The model under review builds one solid part; all positions refer to its coordinate system, in mm. Face numbers are marked on the shaded views. A direction names the side the tool comes from. Coordinates: 2 decimals unless noted, no trailing zeros. Order: outer loops, then holes, each group sorted by start corner. A loop starts at its lowest first (then second) coordinate and runs counter-clockwise, first axis right, second up.
```python
from build123d import *

# Parameters (mm, degrees)
BOSS_EXTRU_1_DEPTH      = 36
ESQUISSE2_W             = 20
ESQUISSE2_H             = 15
BOSS_EXTRU_2_DEPTH      = 4
ESQUISSE3_R             = 3.2
ENL_V_MAT_EXTRU_1_DEPTH = 4
ESQUISSE4_W             = 20
ESQUISSE4_H             = 4
BOSS_EXTRU_3_DEPTH      = 10


with BuildPart() as part:
    # Esquisse1 → Boss.-Extru.1 (new body)
    with BuildSketch(Plane.XY):
        Polygon((0, 0), (-5, 0), (-5, 15), (0, 15), (0, 9), (-3, 9), (-3, 6), (0, 6), (0, 2), (10, 2), (10, 6), (13, 6), (13, 9), (10, 9), (10, 15), (15, 15), (15, 0), (10, 0), align=None)
    extrude(amount=BOSS_EXTRU_1_DEPTH)

    # Esquisse2 → Boss.-Extru.2 (add)
    with BuildSketch(Plane.XY.offset(36)):
        with Locations((5, 7.5)):
            Rectangle(ESQUISSE2_W, ESQUISSE2_H)
    extrude(amount=BOSS_EXTRU_2_DEPTH)

    # Esquisse3 → Enlèv. mat.-Extru.1 (cut)
    with BuildSketch(Plane.XY.offset(40)):
        with Locations((5, 7.5)):
            Circle(ESQUISSE3_R)
    extrude(amount=-ENL_V_MAT_EXTRU_1_DEPTH, mode=Mode.SUBTRACT)

    # Esquisse4 → Boss.-Extru.3 (add)
    with BuildSketch(Plane(origin=(0, 15, 0), x_dir=(1, 0, 0), z_dir=(0, 1, 0))):
        with Locations((5, -38)):
            Rectangle(ESQUISSE4_W, ESQUISSE4_H)
    extrude(amount=BOSS_EXTRU_3_DEPTH)


solid = part.part
```
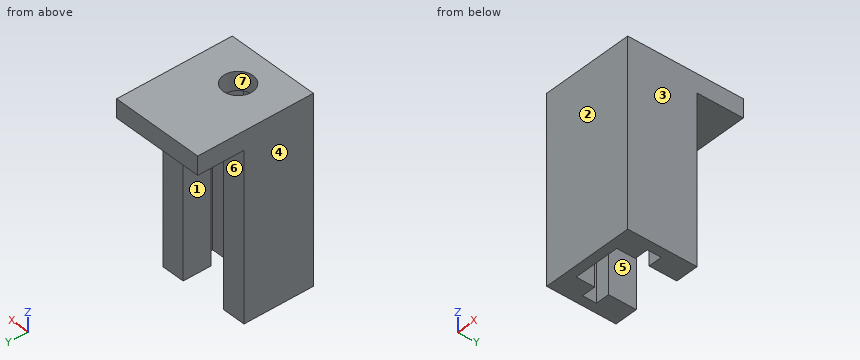
(1) Draft analysis for pull direction X (two halves, no side actions). For the marked faces 1, 2, 3 and 4, state which applies: released by +X, released by -X, zero draft, split by the parting line, or undercut.
A:
face 1: undercut
face 2: zero draft
face 3: released by +X
face 4: released by -X
(2) We need section B-B, the plane y = 7.5. Write out the cut boundary in (x, z), and give its area (3 significant figures).
A:
outline: (-5, 0) - (-3, 0) - (-3, 36) - (1.8, 36) - (1.8, 40) - (-5, 40) - close; (8.2, 36) - (13, 36) - (13, 0) - (15, 0) - (15, 40) - (8.2, 40) - close
area: 198 mm2
(3) Machinability: for the marked faces 5, 6 and 7, which of the approach directions +Z, -Z, +X, -X, +Y, -Y give a long, thin tool a straight path to every point of the face, cutting with its end or side? Answer none if there is none.
A:
face 5: -Z, +Y
face 6: -Z, +X, -X, +Y
face 7: +Z, -Z
(4) We need section D-D, the plane y = 11.75. Write out the cut boundary in (x, z).
A:
outline: (-5, 0) - (0, 0) - (0, 36) - (10, 36) - (10, 0) - (15, 0) - (15, 40) - (-5, 40) - close
(5) We need section C-C, the plane z = 28.5. Write out the cut boundary in (x, y).
A:
outline: (-5, 0) - (15, 0) - (15, 15) - (10, 15) - (10, 9) - (13, 9) - (13, 6) - (10, 6) - (10, 2) - (0, 2) - (0, 6) - (-3, 6) - (-3, 9) - (0, 9) - (0, 15) - (-5, 15) - close
(6) We need section A-A, the plane x = 5. Write out the cut boundary in (y, z).
A:
outline: (0, 0) - (2, 0) - (2, 36) - (4.3, 36) - (4.3, 40) - (0, 40) - close; (10.7, 36) - (25, 36) - (25, 40) - (10.7, 40) - close
(7) For pin 1 Ø3.5 at (x, z) = (-1, 17) entering from +Y; pin 2 Ø3 at (x, y) = (12, 19.5) entering from -Z; pin 3 Ø3 at (x, z) = (3, 25) entering from +Y, all flat-tipped, find the tip position at first contact; note any pin that passes through.
A:
pin 1: stops at y = 15
pin 2: stops at z = 36
pin 3: stops at y = 2
(8) Wall thickness on probe 1 along Y at (x, z) = (5, 37.15); probe 2 along X at (y, z) = (14.75, 33.5); probe 3 along Y at (x, z) = (-2.5, 9): over which ranges is each line inside the solid? List them lowest first.
A:
probe 1: y = 0 to 4.3, 10.7 to 25
probe 2: x = -5 to 0, 10 to 15
probe 3: y = 0 to 6, 9 to 15
